The model under review builds one solid part; all positions refer to its coordinate system, in mm. Face numbers are marked on the shaded views. A direction names the side the tool comes from. Round coordinates to 2 decimals unless told otherwise and drop trailing zeros. Order: outer loops, then holes, each group sorted by start corner. A loop starts at its lowest first (then second) coordinate and runs counter-clockwise, first axis right, second up. Notation, with made-up numbers: M 44.5,3 L 52.5,3 A6 ccw 52.5,7 Z; hole C 71.25,8 d3. An arc over 180 degrees is marked long. Answer as a JSON object with one key per item and string values. Group by question number.
1. Add section A-A on z = 1143. State the section outline as (x, y) points (3 decimals).
2. Add section B-B on y = 22.25. State the section outline as (x, z) points (3 decimals), and give its area (3 significant figures).
3. Machinability: for the marked faces 1 and 2, which of the approach directions +Z, -Z, +X, -X, +Y, -Y give a long, thin tool a straight path to every point of the face, cutting with its end or side? Answer none if there is none.
4. To check wall thickness, follow probe 1 along Y at (x, z) = (12.25, 1124) (3 decimals); probe 2 along Z at (x, y) = (5.75, 2.75). State the ranges of each line that lie inside material, in increasing order. Write a range as [from, to].
5. Clearance check with flat-ended pins moving along their axes: P1, Ø2, axis at x = 19.5, z = 1149.5, coming from the +Y side (3 decimals); P2, Ø3, axis at y = 12, z = 1133.5, coming from the +X side (3 decimals); P3, Ø3.5, axis at x = 1, z = 1025.5, coming from the -Y side (3 decimals). State where each tip first meets the part, or that it passes through.
6. Add section C-C on x = 9.25. State the section outline as (y, z) points (3 decimals).
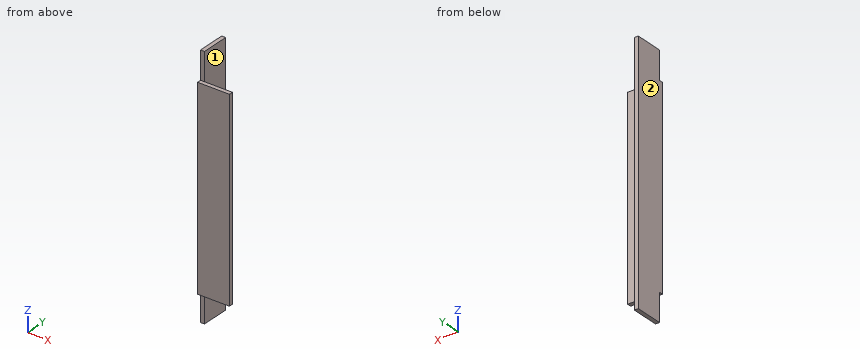
```python
from build123d import *

# Parameters (mm, degrees)
BOSS_EXTRUDE1_DEPTH = 1219.2
FILLET1_R           = 0.4064
SKETCH4_W           = 2238.4
SKETCH4_H           = 103.278519729
CUT_EXTRUDE1_DEPTH  = 60
SKETCH5_W           = 25.4
SKETCH5_H           = 22.23
CUT_EXTRUDE2_DEPTH  = 3.175
SKETCH6_W           = 25.4
SKETCH6_H           = 22.23
CUT_EXTRUDE3_DEPTH  = 3.175
SKETCH7_W           = 1.26890891
SKETCH7_H           = 1.024965533
CUT_EXTRUDE4_DEPTH  = 220


with BuildPart() as part:
    # Sketch3 → Boss-Extrude1 (new, symmetric)
    with BuildSketch(Plane.XY):
        Polygon((3.175, 25.4), (0, 25.4), (0, 0), (25.4, 0), (25.4, 3.175), (3.175, 3.175), align=None)
    extrude(amount=BOSS_EXTRUDE1_DEPTH, both=True)

    # Fillet1
    fillet1_edges = [part.edges().sort_by_distance(p)[0] for p in [
        (3.175, 3.175, 0),
    ]]
    fillet(fillet1_edges, radius=FILLET1_R)

    # Sketch4 → Cut-Extrude1 (cut)
    with BuildSketch(Plane.ZY):
        with Locations((-100, -26.239259864)):
            Rectangle(SKETCH4_W, SKETCH4_H)
    extrude(amount=-CUT_EXTRUDE1_DEPTH, mode=Mode.SUBTRACT)

    # Sketch5 → Cut-Extrude2 (cut)
    with BuildSketch(Plane.XZ):
        with Locations((12.7, 1030.315)):
            Rectangle(SKETCH5_W, SKETCH5_H)
    extrude(amount=-CUT_EXTRUDE2_DEPTH, mode=Mode.SUBTRACT)

    # Sketch6 → Cut-Extrude3 (cut)
    with BuildSketch(Plane.XZ):
        with Locations((12.7, 1208.085)):
            Rectangle(SKETCH6_W, SKETCH6_H)
    extrude(amount=-CUT_EXTRUDE3_DEPTH, mode=Mode.SUBTRACT)

    # Sketch7 → Cut-Extrude4 (cut)
    with BuildSketch(Plane(origin=(0, 0, 1019.2), x_dir=(-1, 0, 0), z_dir=(0, 0, -1))):
        with Locations((-3.809454455, 3.687482767)):
            Rectangle(SKETCH7_W, SKETCH7_H)
    extrude(amount=-CUT_EXTRUDE4_DEPTH, mode=Mode.SUBTRACT)


solid = part.part
```
Recorded:
{
 "1": {"outline": "M 0,0 L 25.4,0 L 25.4,3.175 L 3.175,3.175 L 3.175,25.4 L 0,25.4 Z"},
 "2": {"outline": "M 0,1019.2 L 3.175,1019.2 L 3.175,1219.2 L 0,1219.2 Z", "area": "635 mm²"},
 "3": {"face 1": "+Z, -Z, +X, +Y", "face 2": "+Z, -Z, -X, +Y, -Y"},
 "4": {"probe 1": "y = [0, 3.175]", "probe 2": "z = [1041.43, 1196.97]"},
 "5": {"P1": "stops at y = 3.175", "P2": "stops at x = 3.175", "P3": "stops at y = 3.175"},
 "6": {"outline": "M 0,1041.43 L 3.175,1041.43 L 3.175,1196.97 L 0,1196.97 Z"}
}
